Model file for the job. Use its own axes, mm. Face numbers are marked on the shaded views. A direction names the side the tool comes from. Round coordinates to 2 decimals unless told otherwise and drop trailing zeros. Loops run counter-clockwise (first coordinate to the right, second up) from the corner with the lowest first, then second, coordinate; pieces in that order, holes last. Notation, with made-up numbers: (15.5, 58.25) -> (22.5, 58.25) arc R20 cw to (22.5, 68.25) -> close; hole circle Ø8 at (44, 26.5). An arc over 180 degrees is marked (long way). Use a Markdown table: item, result.
from build123d import *

# Parameters (mm, degrees)
F0_W      = 40
F0_H      = 20
F1_DEPTH  = 4
F2_W      = 20
F2_H      = 20
F3_DEPTH  = 4
F4_W      = 9
F4_H      = 20
F5_DEPTH  = 1
F6_SIZE   = 0.99999
F7_R      = 2.75
F8_DEPTH  = 5.001
F9_SIZE   = 5
F10_R     = 3
F11_DEPTH = 9.001
F13_DEPTH = 2


# Not quite as in the source:
# - a fillet or chamfer is up to 0.001 mm smaller than in the source, because OpenCascade refuses the exact size


with BuildPart() as f1:
    # F0 (on Top) → F1 (new body)
    with BuildSketch(Plane.XY):
        with Locations((20, 10)):
            Rectangle(F0_W, F0_H)
    extrude(amount=F1_DEPTH)

    # F2 (on face) → F3 (join)
    with BuildSketch(Plane.XY.offset(4)):
        with Locations((30, 10)):
            Rectangle(F2_W, F2_H)
    extrude(amount=F3_DEPTH)

    # F4 (on face) → F5 (join)
    with BuildSketch(Plane(origin=(0, 0, 0), x_dir=(1, 0, 0), z_dir=(0, 0, -1))):
        with Locations((10, -10)):
            Rectangle(F4_W, F4_H)
    extrude(amount=F5_DEPTH)

    # F6 (size 1 in the source; OpenCascade refuses exactly that, so slightly less here)
    f6_edges = [f1.edges().sort_by_distance(p)[0] for p in [
        (10, 0, -1),
        (5.5, 10, -1),
        (10, 20, -1),
        (14.5, 10, -1),
    ]]
    chamfer(f6_edges, length=F6_SIZE)

    # F7 (on face) → F8 (cut, through all)
    with BuildSketch(Plane.XY.offset(4)):
        with Locations((10, 10)):
            Circle(F7_R)
    extrude(amount=-F8_DEPTH, mode=Mode.SUBTRACT)

    # F9
    f9_edges = [f1.edges().sort_by_distance(p)[0] for p in [
        (40, 0, 4),
        (40, 20, 4),
        (20, 0, 6),
        (20, 20, 6),
    ]]
    chamfer(f9_edges, length=F9_SIZE)

    # F10 (on face) → F11 (cut, through all)
    with BuildSketch(Plane.XY.offset(8)):
        with Locations((30, 10)):
            Circle(F10_R)
    extrude(amount=-F11_DEPTH, mode=Mode.SUBTRACT)

    # F12 (on face) → F13 (cut, symmetric)
    with BuildSketch(Plane.XY.offset(4)):
        Polygon((25.4389328734, 10), (27.7194664367, 6.05), (40, 6.05), (40, 13.95), (27.7194664367, 13.95), align=None)
    extrude(amount=F13_DEPTH, both=True, mode=Mode.SUBTRACT)


solid = f1.part
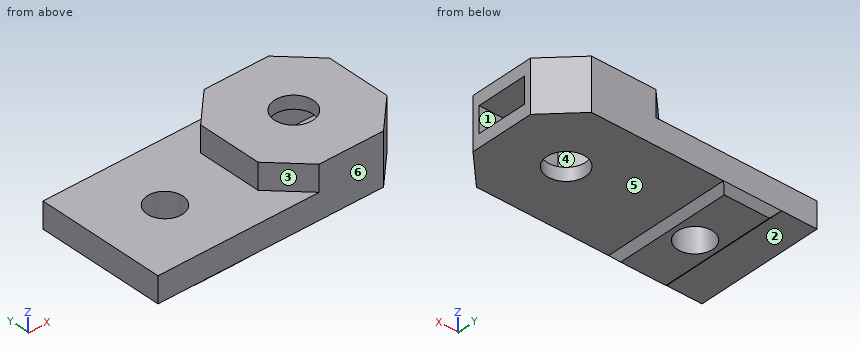
Q1. Band-saw the part on C-C, the plane y = 12.25. Give the number of separate pieces and of enclosed holes in the cut face, plus the area to 3 significant figures.
Results list:
| item | result |
|---|---|
| separate pieces | 4 |
| enclosed holes | 0 |
| area | 163 mm² |
Q2. Band-saw the part on A-A, the plane x = 30. Give the cut face in (y, z), plus the area to 3 significant figures.
Results list:
| item | result |
|---|---|
| outline | (0, 0) -> (7, 0) -> (7, 2) -> (6.05, 2) -> (6.05, 6) -> (7, 6) -> (7, 8) -> (0, 8) -> close; (13, 0) -> (20, 0) -> (20, 8) -> (13, 8) -> (13, 6) -> (13.95, 6) -> (13.95, 2) -> (13, 2) -> close |
| area | 104 mm² |
Q3. Drill centre lines: L1, parallel to Y at x = 30, z = 0.6; L2, parallel to Y at x = 10, z = 2.6; L3, parallel to Z at x = 32.5, y = 11.75. Where is each one in solid material? Low to high. Write a range as from..to.
Results list:
| item | result |
|---|---|
| L1 | y = 0..7, 13..20 |
| L2 | y = 0..7.25, 12.75..20 |
| L3 | z = 0..2, 6..8 |
Q4. Flat gauge pins, fed straight in: pin 1 (7 mm diameter, centred on x = 30, y = 10, fed in from +Z); pin 2 (10 mm diameter, centred on x = 13.5, y = 13, fed in from +Z). Where does each tip first touch, or does it go through?
Results list:
| item | result |
|---|---|
| pin 1 | stops at z = 8 |
| pin 2 | stops at z = 4 |
Q5. Band-saw the part on B-B, the plane z = 1.25. Give the cut face in (x, y), plus the area to 3 significant figures.
Results list:
| item | result |
|---|---|
| outline | (0, 0) -> (35, 0) -> (40, 5) -> (40, 15) -> (35, 20) -> (0, 20) -> close; hole circle Ø5.5 at (10, 10); hole circle Ø6 at (30, 10) |
| area | 723 mm² |
Q6. Pull direction Z, two halves, no side cores. Call the marked faces 4, 5 and 6: released by +Z, released by -Z, zero draft, split by the parting line, or undercut.
Results list:
| item | result |
|---|---|
| face 4 | undercut |
| face 5 | released by -Z |
| face 6 | zero draft |
Q7. Band-saw the part on D-D, the plane x = 37.5. Give the cut face in (y, z).
Results list:
| item | result |
|---|---|
| outline | (2.5, 0) -> (17.5, 0) -> (17.5, 8) -> (2.5, 8) -> close; hole (6.05, 2) -> (13.95, 2) -> (13.95, 6) -> (6.05, 6) -> close |
Q8. Tool access for the marked faces 1, 2 and 3: list every direction of +Z, -Z, +X, -X, +Y, -Y with a clear straight run to the whole face (end or side of a thin tool).
Results list:
| item | result |
|---|---|
| face 1 | +X |
| face 2 | -Z, -X, +Y, -Y |
| face 3 | +Z, -X, -Y |
